Source: three-view drawing plus pictorial views. Frame: mm from the lowest corner of the part. Round coordinates to 2 decimals unless told otherwise and drop trailing zeros. Write each loop counter-clockwise with the first axis right and the second up, starting at its lowest first coordinate (ties: lowest second). Pieces come first, ordered by that corner, then holes. Notation, with made-up numbers: (11.5, 69) -> (61.5, 69) arc R30 ccw to (61.5, 107) -> close; hole circle Ø9 at (76.5, 82.25). An arc over 180 degrees is marked (long way). Put each result on its own line as item: value.
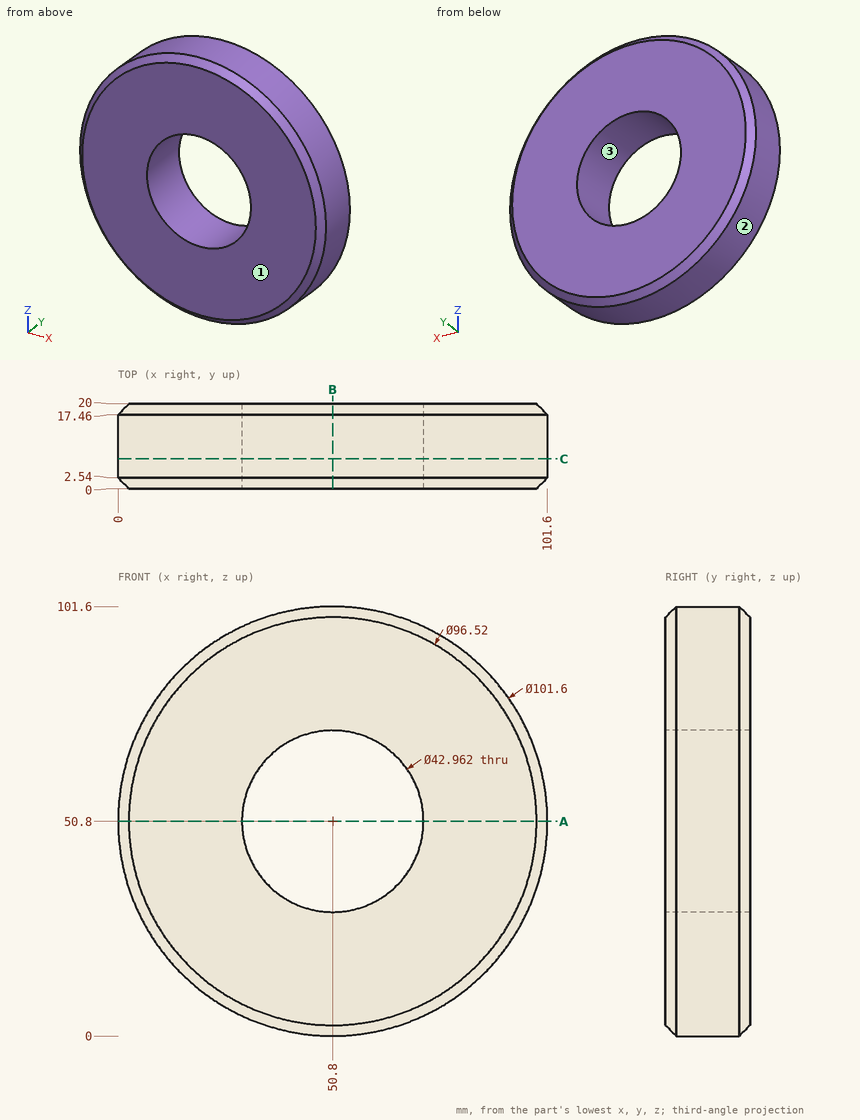
Q1. Material intervals for line 1 (Z direction, x = 50.8, y = 15); line 2 (Z direction, x = 66.5, y = 10.5) (1 decimal); line 3 (X direction, y = 6.5, z = 63.5) (1 decimal), sorted ascending. Write a range as [from, to].
Ans:
line 1: z = [0, 29.32], [72.28, 101.6]
line 2: z = [2.5, 36.1], [65.5, 99.1]
line 3: x = [1.6, 33.5], [68.1, 100]
Q2. Cut plane C-C on y = 7. Output: boundary loops of the cut face in (x, z), and give its area (3 significant figures).
Ans:
outline: circle Ø101.6 at (50.8, 50.8); hole circle Ø42.96 at (50.8, 50.8)
area: 6,660 mm^2
Q3. Draft query along Z for the marked faces 1, 2 and 3. Return one class per face: +Z half, -Z half, draft (parallel to the pull), parting line (faces both ways), or undercut.
Ans:
face 1: draft
face 2: parting line
face 3: undercut
Q4. Pin query (flat end, axial travel): pin 1 (5 mm diameter, centred on x = 55.5, y = 15.5, fed in from -Z); pin 2 (6 mm diameter, centred on y = 17.5, z = 73, fed in from +X); pin 3 (1.5 mm diameter, centred on x = 59, y = 13, fed in from -Z). Return the tip coordinate at first contact, or that it passes through.
Ans:
pin 1: stops at z = 0.05
pin 2: stops at x = 97.83
pin 3: stops at z = 0.55
Q5. Cut plane B-B on x = 50.8. Output: boundary loops of the cut face in (y, z).
Ans:
outline: (0, 2.54) -> (2.54, 0) -> (17.46, 0) -> (20, 2.54) -> (20, 29.32) -> (0, 29.32) -> close; (0, 72.28) -> (20, 72.28) -> (20, 99.06) -> (17.46, 101.6) -> (2.54, 101.6) -> (0, 99.06) -> close
Q6. Cut plane A-A on z = 50.8. Output: boundary loops of the cut face in (x, y).
Ans:
outline: (0, 2.54) -> (2.54, 0) -> (29.32, 0) -> (29.32, 20) -> (2.54, 20) -> (0, 17.46) -> close; (72.28, 0) -> (99.06, 0) -> (101.6, 2.54) -> (101.6, 17.46) -> (99.06, 20) -> (72.28, 20) -> close
